Can you work these out from the drawing? Everything is in mm from the part's minimum corner. Coordinates: 2 decimals unless noted, no trailing zeros. Write each loop counter-clockwise with the first axis right and the second up, starting at its lowest first coordinate (ties: lowest second). Pieces come first, ordered by that corner, then holes. Notation, with made-up numbers: (-22, -32.75) -> (32, -32.75) arc R13 cw to (32, -15.75) -> close; hole circle Ø5 at (53.25, -3). An arc over 180 degrees is marked (long way). Use a Markdown table: item, result. Add a question column.
Item 1: If I drill on line 1 along Z through (x, y) = (1.75, 10); line 2 along Z through (x, y) = (1.45, 14.5); line 3 along Y through (x, z) = (2.3, 44.5) (3 decimals), over which ranges is the centre line in solid material (lowest first)? Write a range as from..to.
Item 2: Imagine slicing it at A-A, the plane y = 10.5. Write out the boundary of the cut face in (x, z).
Item 3: Imagine slicing it at C-C, the plane z = 44. Write out the boundary of the cut face in (x, y).
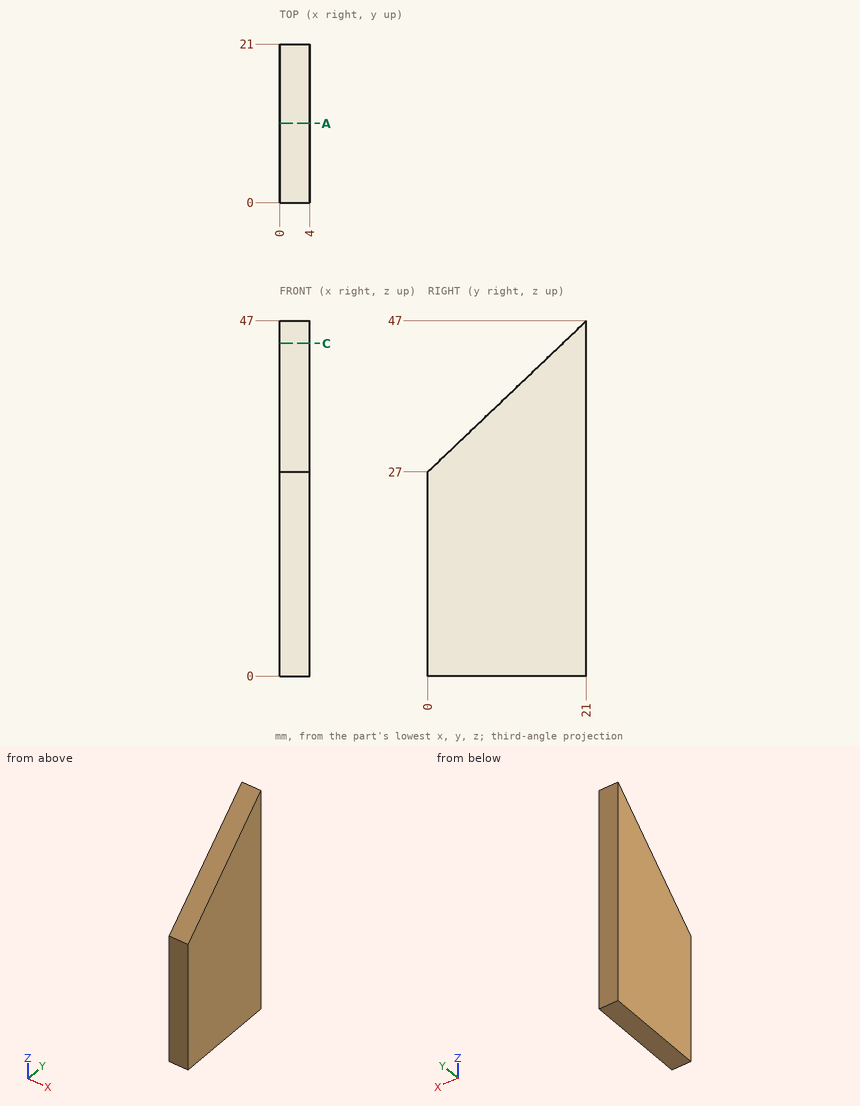
Ans:
| question | item | result |
|---|---|---|
| 1 | line 1 | z = 0..36.52 |
| 1 | line 2 | z = 0..40.81 |
| 1 | line 3 | y = 18.375..21 |
| 2 | outline | (0, 0) -> (4, 0) -> (4, 37) -> (0, 37) -> close |
| 3 | outline | (0, 17.85) -> (4, 17.85) -> (4, 21) -> (0, 21) -> close |
